Input: dimensioned drawing with shaded views. Units: mm. Origin: part minimum x, y, z. A direction names the side the tool comes from. Give positions to 0.01 mm unless a question says otherwise; leave off trailing zeros. Write each loop counter-clockwise with the first axis right and the second up, starting at its lowest first coordinate (ties: lowest second). Pieces come first, ordered by that corner, then holes. Notation, with made-up numbers: M 60,5.25 L 88,5.25 A20 ccw 88,13.25 Z; hole C 6,62.25 d4. An arc over 180 degrees is marked long. Answer as a JSON object with one key per item and string values.
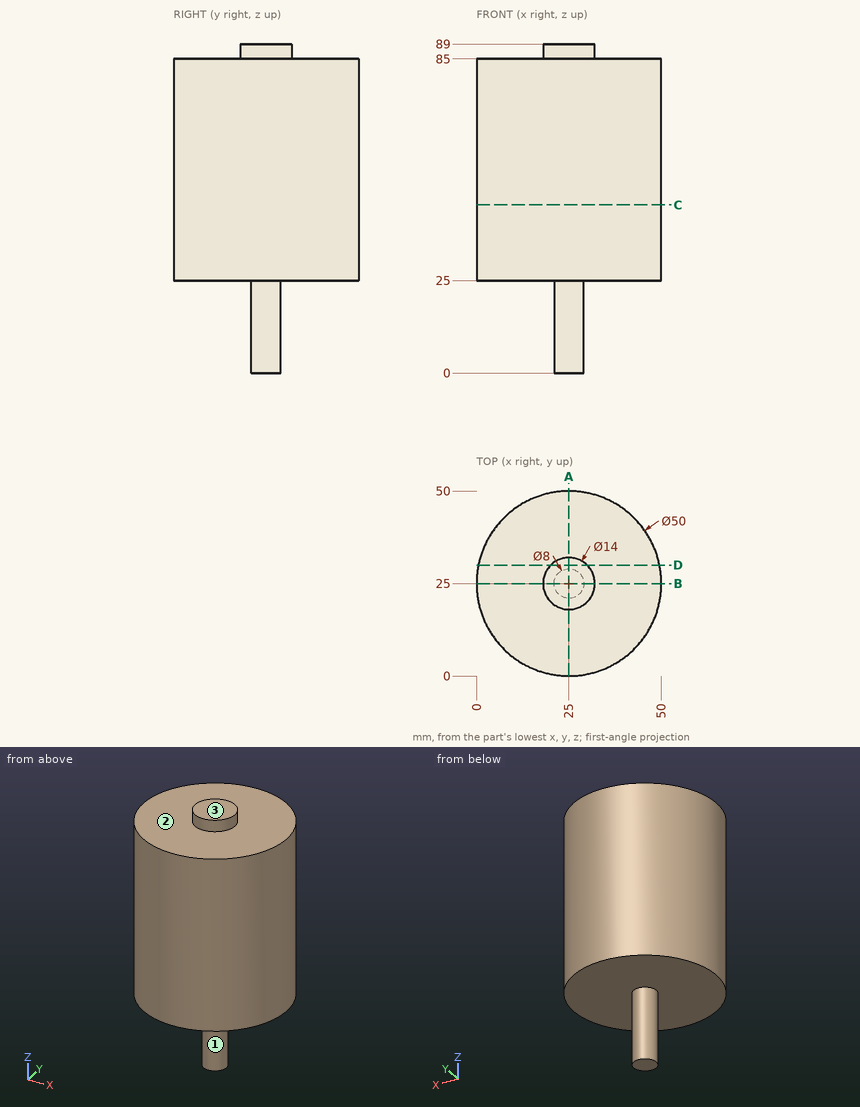
1) Cut plane C-C on z = 45.5. Return loops of the section in (x, y), and give its area (3 significant figures).
Geometry check:
{"outline": "C 25,25 d50", "area": "1,960 mm2"}
2) Cut plane D-D on y = 30. Return loops of the section in (x, z).
Geometry check:
{"outline": "M 0.51,25 L 49.49,25 L 49.49,85 L 29.9,85 L 29.9,89 L 20.1,89 L 20.1,85 L 0.51,85 Z"}
3) Contact query for flat-ended pins moving along their axis: P1, Ø3, axis at x = 40, z = 58.5, coming from the -Y side; P2, Ø8, axis at x = 14, z = 68.5, coming from the -Y side; P3, Ø10, axis at x = 40, z = 17.5, coming from the +Y side; P4, Ø4, axis at y = 12, z = 45, coming from the +X side. Output: stop coordinate, or through.
Geometry check:
{"P1": "stops at y = 3.96", "P2": "stops at y = 1", "P3": "passes through", "P4": "stops at x = 47.45"}
4) Cut plane A-A on x = 25. Return loops of the section in (y, z), and give its area (3 significant figures).
Geometry check:
{"outline": "M 0,25 L 21,25 L 21,0 L 29,0 L 29,25 L 50,25 L 50,85 L 32,85 L 32,89 L 18,89 L 18,85 L 0,85 Z", "area": "3,260 mm2"}
5) Line query: line 1 (Z direction, x = 23.5, y = 4); line 2 (X direction, y = 24.5, z = 26.5) (3 decimals); line 3 (Y direction, x = 34.5, z = 72.5). Output: solid intervals per line, ascending. Write a range as from..to.
Geometry check:
{"line 1": "z = 25..85", "line 2": "x = 0.005..49.995", "line 3": "y = 1.88..48.12"}
6) Set-up query: the marked faces 1, 2 and 3. Return all of +Z, -Z, +X, -X, +Y, -Y with unobstructed straight access to the full face (end or side cutting, diameter ignored); none if empty.
Geometry check:
{"face 1": "-Z", "face 2": "+Z", "face 3": "+Z, +X, -X, +Y, -Y"}
